Verification items for the finished model (mm, model axes). A direction names the side the tool comes from. Round coordinates to 2 decimals unless told otherwise and drop trailing zeros. Write each loop counter-clockwise with the first axis right and the second up, starting at its lowest first coordinate (ties: lowest second). Pieces come first, ordered by that corner, then holes. Notation, with made-up numbers: M 9.5,-30.5 L 18.5,-30.5 A32 cw 18.5,8.5 Z; hole C -26.75,14.5 d11. An arc over 180 degrees is marked long. One line per item, written item: value. Start each with the question number.
from build123d import *

# Parameters (mm, degrees)
F0_W      = 25
F0_H      = 30
F0_R      = 9.25
F0_W_2    = 3
F1_DEPTH  = 5
F2_DEPTH  = 40
F3_R      = 10
F4_R      = 1.75
F5_DEPTH  = 3.001
F7_DEPTH  = 30
F8_W      = 32.9495297466
F8_H      = 1.9953548908
F8_H_2    = 2.0693931729
F8_H_3    = 2.1812524647
F8_H_4    = 2.4609006941
F8_H_5    = 1.9016051665
F8_H_6    = 1.9016047008
F8_H_7    = 1.454168465
F8_H_8    = 1.1185912881
F9_DEPTH  = 18.69
F11_DEPTH = 30.001
F13_DEPTH = 30


with BuildPart() as f1:
    # F0 (on Top) → F1 (new body)
    with BuildSketch(Plane.XY):
        with Locations((-12.5, 15)):
            Rectangle(F0_W, F0_H)
        with Locations((-12, 15)):
            Circle(F0_R, mode=Mode.SUBTRACT)
        with Locations((-26.5, 15)):
            Rectangle(F0_W_2, F0_H)
    extrude(amount=F1_DEPTH)

    # F0 (on Top) → F2 (join)
    with BuildSketch(Plane.XY):
        with Locations((-26.5, 15)):
            Rectangle(F0_W_2, F0_H)
    extrude(amount=F2_DEPTH)

    # F3
    f3_edges = [f1.edges().sort_by_distance(p)[0] for p in [
        (0, 0, 2.5),
        (0, 30, 2.5),
    ]]
    fillet(f3_edges, radius=F3_R)

    # F4 (on face) → F5 (cut, through all)
    with BuildSketch(Plane.YZ.offset(-25)):
        with Locations((5, 32.5)):
            Circle(F4_R)
        with BuildLine():
            ThreePointArc((25.8762976423, 34.0147945214), (26.5159190074, 33.3743509381), (26.75, 32.5))
            ThreePointArc((26.75, 32.5), (26.5151696279, 31.6243510986), (25.8737017159, 30.9837067198))
            ThreePointArc((25.8737017159, 30.9837067198), (26.2572446424, 30.8193071518), (26.6688053839, 30.7503858164))
            Line((26.6688053839, 30.7503858164), (26.8316769531, 30.7504083459))
            ThreePointArc((26.8316769531, 30.7504083459), (28.015984309, 31.290286813), (28.4999993582, 32.4985012412))
            ThreePointArc((28.4999993582, 32.4985012412), (27.9856735638, 33.7376982625), (26.7450173494, 34.2484941496))
            ThreePointArc((26.7450173494, 34.2484941496), (26.2953839701, 34.1884198336), (25.8762976423, 34.0147945214))
        make_face()
        with BuildLine():
            ThreePointArc((25.313264961, 33.4976480132), (25.5661966357, 33.7873422376), (25.8762976423, 34.0147945214))
            ThreePointArc((25.8762976423, 34.0147945214), (25.5235901108, 34.1698363381), (25.1455039627, 34.2439405371))
            Line((25.1455039627, 34.2439405371), (24.8445689194, 34.243083813))
            ThreePointArc((24.8445689194, 34.243083813), (24.6385972754, 34.2122756994), (24.4377440921, 34.1572170329))
            ThreePointArc((24.4377440921, 34.1572170329), (24.9284794863, 33.8977522036), (25.313264961, 33.4976480132))
        make_face()
        with BuildLine():
            ThreePointArc((25.1455039627, 34.2439405371), (25.5235901108, 34.1698363381), (25.8762976423, 34.0147945214))
            ThreePointArc((25.8762976423, 34.0147945214), (26.2953839701, 34.1884198336), (26.7450173494, 34.2484941496))
            Line((26.7450173494, 34.2484941496), (25.1455039627, 34.2439405371))
        make_face()
        with BuildLine():
            ThreePointArc((26.6688053839, 30.7503858164), (26.2572446424, 30.8193071518), (25.8737017159, 30.9837067198))
            ThreePointArc((25.8737017159, 30.9837067198), (25.4635661352, 30.8125147591), (25.0235325622, 30.7501582304))
            Line((25.0235325622, 30.7501582304), (26.6688053839, 30.7503858164))
        make_face()
        with BuildLine():
            ThreePointArc((25.0235325622, 30.7501582304), (25.4635661352, 30.8125147591), (25.8737017159, 30.9837067198))
            ThreePointArc((25.8737017159, 30.9837067198), (25.5644222061, 31.2112923163), (25.3122242271, 31.5008526697))
            ThreePointArc((25.3122242271, 31.5008526697), (24.927751526, 31.1016985717), (24.4377457378, 30.8427824088))
            ThreePointArc((24.4377457378, 30.8427824088), (24.7037063498, 30.7752652167), (24.97695154, 30.750151787))
            Line((24.97695154, 30.750151787), (25.0235325622, 30.7501582304))
        make_face()
        with BuildLine():
            Line((24.8445689194, 34.243083813), (25.1455039627, 34.2439405371))
            ThreePointArc((25.1455039627, 34.2439405371), (24.9950179912, 34.2499929084), (24.8445689194, 34.243083813))
        make_face()
        with BuildLine():
            ThreePointArc((24.97695154, 30.750151787), (25.0002420726, 30.7500000167), (25.0235325622, 30.7501582304))
            Line((25.0235325622, 30.7501582304), (24.97695154, 30.750151787))
        make_face()
        with BuildLine():
            Line((26.8316769531, 30.7504083459), (26.6688053839, 30.7503858164))
            ThreePointArc((26.6688053839, 30.7503858164), (26.7502414308, 30.7485012579), (26.8316769531, 30.7504083459))
        make_face()
        with BuildLine():
            ThreePointArc((24.4377440921, 34.1572170329), (24.6385972754, 34.2122756994), (24.8445689194, 34.243083813))
            Line((24.8445689194, 34.243083813), (24.0543595868, 34.2408341869))
            ThreePointArc((24.0543595868, 34.2408341869), (24.248402903, 34.2098052318), (24.4377440921, 34.1572170329))
        make_face()
        with BuildLine():
            ThreePointArc((24.4377457378, 30.8427824088), (23.25, 32.4999991311), (24.4377440921, 34.1572170329))
            ThreePointArc((24.4377440921, 34.1572170329), (24.248402903, 34.2098052318), (24.0543595868, 34.2408341869))
            Line((24.0543595868, 34.2408341869), (23.6867111794, 34.2397875383))
            ThreePointArc((23.6867111794, 34.2397875383), (22.1280512127, 32.4053512558), (23.8757319025, 30.7499994584))
            ThreePointArc((23.8757319025, 30.7499994584), (24.1605392352, 30.7733706928), (24.4377457378, 30.8427824088))
        make_face()
        with BuildLine():
            Line((23.8757319025, 30.7499994584), (24.97695154, 30.750151787))
            ThreePointArc((24.97695154, 30.750151787), (24.7037063498, 30.7752652167), (24.4377457378, 30.8427824088))
            ThreePointArc((24.4377457378, 30.8427824088), (24.1605392352, 30.7733706928), (23.8757319025, 30.7499994584))
        make_face()
        with BuildLine():
            Line((23.6867111794, 34.2397875383), (24.0543595868, 34.2408341869))
            ThreePointArc((24.0543595868, 34.2408341869), (23.8705078211, 34.2499923501), (23.6867111794, 34.2397875383))
        make_face()
        with BuildLine():
            ThreePointArc((25.8737017159, 30.9837067198), (26.5151696279, 31.6243510986), (26.75, 32.5))
            ThreePointArc((26.75, 32.5), (26.5159190074, 33.3743509381), (25.8762976423, 34.0147945214))
            ThreePointArc((25.8762976423, 34.0147945214), (25.5661966357, 33.7873422376), (25.313264961, 33.4976480132))
            ThreePointArc((25.313264961, 33.4976480132), (25.545610556, 33.0226817163), (25.6254898299, 32.4999994417))
            ThreePointArc((25.6254898299, 32.4999994417), (25.5453379061, 31.9764467676), (25.3122242271, 31.5008526697))
            ThreePointArc((25.3122242271, 31.5008526697), (25.5644222061, 31.2112923163), (25.8737017159, 30.9837067198))
        make_face()
        with BuildLine():
            ThreePointArc((25.3122242271, 31.5008526697), (24.9999995959, 32.4994133448), (25.313264961, 33.4976480132))
            ThreePointArc((25.313264961, 33.4976480132), (24.9284794863, 33.8977522036), (24.4377440921, 34.1572170329))
            ThreePointArc((24.4377440921, 34.1572170329), (23.25, 32.4999991311), (24.4377457378, 30.8427824088))
            ThreePointArc((24.4377457378, 30.8427824088), (24.927751526, 31.1016985717), (25.3122242271, 31.5008526697))
        make_face()
        with BuildLine():
            ThreePointArc((25.6254898299, 32.4999994417), (25.545610556, 33.0226817163), (25.313264961, 33.4976480132))
            ThreePointArc((25.313264961, 33.4976480132), (24.9999995959, 32.4994133448), (25.3122242271, 31.5008526697))
            ThreePointArc((25.3122242271, 31.5008526697), (25.5453379061, 31.9764467676), (25.6254898299, 32.4999994417))
        make_face()
    extrude(amount=-F5_DEPTH, mode=Mode.SUBTRACT)

    # F6 (on Front) → F7 (join)
    with BuildSketch(Plane.XZ):
        Polygon((-25.9058196098, 40.9654118121), (-39.5162117863, 51.9557070245), (-41.0396176132, 50.6510883904), (-28.0414205045, 39.976708591), (-25.5407467018, 39.976708591), align=None)
        Polygon((-29.4997693367, 60.5336166234), (-30.6862313423, 62.3977148942), (-55.7127751532, 40.9654118121), (-54.2898289063, 39.3038345914), (-41.0396176132, 50.6510883904), (-39.5162117863, 51.9557070245), align=None)
    extrude(amount=-F7_DEPTH)

    # F8 (on face) → F9 (cut)
    with BuildSketch(Plane(origin=(-43.8108490147, 0, 51.1580173188), x_dir=(0.7595417599, 0, 0.6504585421), z_dir=(-0.6504585421, 0, 0.7595417599))):
        with Locations((0.8048876299, 27.0703136921)):
            Rectangle(F8_W, F8_H)
        with Locations((0.8048876299, 22.6615490392)):
            Rectangle(F8_W, F8_H_2)
        with Locations((0.8048876299, 18.6346201226)):
            Rectangle(F8_W, F8_H_3)
        with Locations((0.8048876299, 14.3560096622)):
            Rectangle(F8_W, F8_H_4)
        with Locations((0.8048876299, 10.2172228508)):
            Rectangle(F8_W, F8_H_5)
        with Locations((0.8048876299, 7.0292379241)):
            Rectangle(F8_W, F8_H_6)
        with Locations((0.8048876299, 3.7853235845)):
            Rectangle(F8_W, F8_H_7)
        with Locations((0.8048876299, 1.5481411247)):
            Rectangle(F8_W, F8_H_8)
    extrude(amount=-F9_DEPTH, mode=Mode.SUBTRACT)

    # F10 (on face) → F11 (cut, through all)
    with BuildSketch(Plane(origin=(0, 30, 0), x_dir=(-1, 0, 0), z_dir=(0, 1, 0))):
        Polygon((32.9848708997, 57.549035391), (30.6862313423, 62.3977148942), (29.4997693367, 60.5336166234), align=None)
        Polygon((50.0453349621, 42.9387464406), (54.2898289063, 39.3038345914), (55.7127751532, 40.9654118121), align=None)
    extrude(amount=-F11_DEPTH, mode=Mode.SUBTRACT)

    # F12 (on Front) → F13 (join)
    with BuildSketch(Plane.XZ):
        Polygon((-24.968046695, 20.0552176684), (-24.968046695, 5.0357975997), (-16.1222536117, 4.974368494), align=None)
    extrude(amount=F13_DEPTH)


solid = f1.part
1) Mould release check, pull along Z, two halves, no side actions. Record for faces 1 (the flat face through (-45.606, 8.614, 46.741)), 2 (the flat face through (-23, -30, 9)), 3 (the flat face through (-31.85, 0.5, 59.94)): pulls with the +Z half, pulls with the -Z half, needs draft (parallel to the pull), parting line crosses it, or undercut.
2) Thickness scan on line 1 (X direction, y = 5, z = 21.5); line 2 (Z direction, x = -8, y = 4); line 3 (Y direction, x = -12, z = 2). Record the ranges inside material, lowest first.
3) Cross-section at B-B (z = 8). Record the boundary of the cut face in (x, y), then the cut area to 3 significant figures.
4) Access from +Z, -Z, +X, -X, +Y, -Y to the whole of each face (thin tool, end or side, straight path). Record for faces 4 (the flat face through (-31.85, 24.9, 59.94)), 5 (the flat face through (-52.919, 12.16, 41.938)), 6 (the flat face through (-27.285, 27.084, 40.704)).
5) Cross-section at A-A (x = -7). Record the boundary of the cut face in (y, z), then the cut area to 3 significant figures.
6) Gauge pin test, flat ends, axial feed: pin 1 Ø18 at (x, z) = (-39.5, 51.5) entering from -Y; pin 2 Ø3 at (y, z) = (5, 32.5) entering from +X; pin 3 Ø1.5 at (y, z) = (4.5, 20) entering from -X; pin 4 Ø20 at (x, y) = (-12.5, 15) entering from +Z. Record the tip position at first contact, or that the pin passes through.
7) Cross-section at D-D (x = -42.5). State how many separate pieces and enclosed holes the cut face has, then the cut area to 3 significant figures.
8) Cross-section at C-C (y = -3.5). Record the boundary of the cut face in (x, z).
Results below:
1. face 1: pulls with the -Z half
1. face 2: needs draft
1. face 3: undercut
2. line 1: x = -28 to -25
2. line 2: z = 0 to 5
2. line 3: y = 0 to 5.75, 24.25 to 30
3. outline: M -28,0 L -25,0 L -25,30 L -28,30 Z; M -24.97,-30 L -17.9,-30 L -17.9,0 L -24.97,0 Z
3. area: 302 mm²
4. face 4: +X, +Y, -Y
4. face 5: -Z, +Y, -Y
4. face 6: +Z, -X
5. outline: M 0.46,0 L 7.22,0 L 7.22,5 L 0.46,5 Z; M 22.78,0 L 29.54,0 L 29.54,5 L 22.78,5 Z
5. area: 67.6 mm²
6. pin 1: stops at y = 0
6. pin 2: passes through
6. pin 3: stops at x = -28
6. pin 4: stops at z = 5
7. separate pieces: 9
7. enclosed holes: 0
7. area: 43.0 mm²
8. outline: M -24.97,5.04 L -16.12,4.97 L -24.97,20.06 Z
